```python
from build123d import *

# Parameters (mm, degrees)
F0_R     = 3.175
F1_DEPTH = 25.4


with BuildPart() as f1:
    # F0 (on Top) → F1 (new body)
    with BuildSketch(Plane.XY):
        with BuildLine():
            ThreePointArc((6.2681930411, -1.016), (6.3295152188, -0.5096440862), (6.35, 0))
            ThreePointArc((6.35, 0), (6.3295152188, 0.5096440862), (6.2681930411, 1.016))
            Line((6.2681930411, 1.016), (5.7634121265, 1.016))
            Line((5.7634121265, 1.016), (5.176824253, 0))
            Line((5.176824253, 0), (5.7634121265, -1.016))
            Line((5.7634121265, -1.016), (6.2681930411, -1.016))
        make_face()
        with BuildLine():
            ThreePointArc((6.2681930411, 1.016), (6.3295152188, 0.5096440862), (6.35, 0))
            ThreePointArc((6.35, 0), (6.3295152188, -0.5096440862), (6.2681930411, -1.016))
            Line((6.2681930411, -1.016), (6.9365878735, -1.016))
            Line((6.9365878735, -1.016), (7.523175747, 0))
            Line((7.523175747, 0), (6.9365878735, 1.016))
            Line((6.9365878735, 1.016), (6.2681930411, 1.016))
        make_face()
        with BuildLine():
            Line((5.7634121265, 1.016), (6.2681930411, 1.016))
            ThreePointArc((6.2681930411, 1.016), (4.4901280605, 4.4901280605), (1.016, 6.2681930411))
            Line((1.016, 6.2681930411), (1.016, 5.7634121265))
            Line((1.016, 5.7634121265), (0, 5.176824253))
            Line((0, 5.176824253), (-1.016, 5.7634121265))
            Line((-1.016, 5.7634121265), (-1.016, 6.2681930411))
            ThreePointArc((-1.016, 6.2681930411), (-4.4901280605, 4.4901280605), (-6.2681930411, 1.016))
            Line((-6.2681930411, 1.016), (-5.7634121265, 1.016))
            Line((-5.7634121265, 1.016), (-5.176824253, 0))
            Line((-5.176824253, 0), (-5.7634121265, -1.016))
            Line((-5.7634121265, -1.016), (-6.2681930411, -1.016))
            ThreePointArc((-6.2681930411, -1.016), (-4.4901280605, -4.4901280605), (-1.016, -6.2681930411))
            Line((-1.016, -6.2681930411), (-1.016, -5.7634121265))
            Line((-1.016, -5.7634121265), (0, -5.176824253))
            Line((0, -5.176824253), (1.016, -5.7634121265))
            Line((1.016, -5.7634121265), (1.016, -6.2681930411))
            ThreePointArc((1.016, -6.2681930411), (4.4901280605, -4.4901280605), (6.2681930411, -1.016))
            Line((6.2681930411, -1.016), (5.7634121265, -1.016))
            Line((5.7634121265, -1.016), (5.176824253, 0))
            Line((5.176824253, 0), (5.7634121265, 1.016))
        make_face()
        Circle(F0_R, mode=Mode.SUBTRACT)
        with BuildLine():
            Line((1.016, 5.7634121265), (1.016, 6.2681930411))
            ThreePointArc((1.016, 6.2681930411), (0, 6.35), (-1.016, 6.2681930411))
            Line((-1.016, 6.2681930411), (-1.016, 5.7634121265))
            Line((-1.016, 5.7634121265), (0, 5.176824253))
            Line((0, 5.176824253), (1.016, 5.7634121265))
        make_face()
        with BuildLine():
            ThreePointArc((-1.016, 6.2681930411), (0, 6.35), (1.016, 6.2681930411))
            Line((1.016, 6.2681930411), (1.016, 6.9365878735))
            Line((1.016, 6.9365878735), (0, 7.523175747))
            Line((0, 7.523175747), (-1.016, 6.9365878735))
            Line((-1.016, 6.9365878735), (-1.016, 6.2681930411))
        make_face()
        with BuildLine():
            Line((1.016, -6.9365878735), (1.016, -6.2681930411))
            ThreePointArc((1.016, -6.2681930411), (0, -6.35), (-1.016, -6.2681930411))
            Line((-1.016, -6.2681930411), (-1.016, -6.9365878735))
            Line((-1.016, -6.9365878735), (0, -7.523175747))
            Line((0, -7.523175747), (1.016, -6.9365878735))
        make_face()
        with BuildLine():
            ThreePointArc((-1.016, -6.2681930411), (0, -6.35), (1.016, -6.2681930411))
            Line((1.016, -6.2681930411), (1.016, -5.7634121265))
            Line((1.016, -5.7634121265), (0, -5.176824253))
            Line((0, -5.176824253), (-1.016, -5.7634121265))
            Line((-1.016, -5.7634121265), (-1.016, -6.2681930411))
        make_face()
        with BuildLine():
            Line((-5.7634121265, 1.016), (-6.2681930411, 1.016))
            ThreePointArc((-6.2681930411, 1.016), (-6.35, 0), (-6.2681930411, -1.016))
            Line((-6.2681930411, -1.016), (-5.7634121265, -1.016))
            Line((-5.7634121265, -1.016), (-5.176824253, 0))
            Line((-5.176824253, 0), (-5.7634121265, 1.016))
        make_face()
        with BuildLine():
            ThreePointArc((-6.2681930411, -1.016), (-6.35, 0), (-6.2681930411, 1.016))
            Line((-6.2681930411, 1.016), (-6.9365878735, 1.016))
            Line((-6.9365878735, 1.016), (-7.523175747, 0))
            Line((-7.523175747, 0), (-6.9365878735, -1.016))
            Line((-6.9365878735, -1.016), (-6.2681930411, -1.016))
        make_face()
    extrude(amount=F1_DEPTH)


solid = f1.part
```
Verification items for the finished model (mm, model axes). Round coordinates to 2 decimals unless told otherwise and drop trailing zeros. Order: outer loops, then holes, each group sorted by start corner. A loop starts at its lowest first (then second) coordinate and runs counter-clockwise, first axis right, second up. Notation, with made-up numbers: (16, 82) - (27, 82) arc R12 ccw to (27, 88) - close; hole circle Ø11 at (-15, 52). An arc over 180 degrees is marked (long way). Use CSV: the item, a comma, the result in double quotes. Start each with the question number.
1) Mould release check, pull along Y, two halves, no side actions. Record for faces 1 (the cylindrical face through (-0.69, -3.1, 12.52)), 2 (the flat face through (7.234, 0.501, 12.522)), 3 (the cylindrical face through (4.45, -4.53, 12.52)), 4 (the flat face through (-3.4, 0.1, 0)): +Y half, -Y half, draft (parallel to the pull), parting line (faces both ways), or undercut.
2) Thickness scan on L1, parallel to X at y = -2.5, z = 19; L2, parallel to Y at x = -1.5, z = 17.75; L3, parallel to X at y = -1.25, z = 18. Record the ranges inside material, lowest first.
3) Go/stop test with flat-tipped pins: P1, Ø6, axis at x = -3, y = -1.5, coming from the -Z side; P2, Ø3, axis at y = 2, z = 12, coming from the -X side; P3, Ø5, axis at x = -4.5, z = 9, coming from the +Y side; P4, Ø5, axis at y = 5.5, z = 12.5, coming from the +X side. Record where each tip stops, or that it passes through.
4) Section check A-A, the plane z = 3.5. Record the cut outline in (x, y) (3 decimals).
5) Section check D-D, the plane y = 5.75. Record the cut outline in (x, z).
6) Section check C-C, the plane y = -2.75. Record the cut outline in (x, z), plus the area to 3 significant figures.
7) Section check B-B, the plane x = 2.25. Record the cut outline in (y, z), plus the area to 3 significant figures.
Answers:
1,face 1,"undercut"
1,face 2,"+Y half"
1,face 3,"-Y half"
1,face 4,"draft"
2,L1,"x = -5.84 to -1.96, 1.96 to 5.84"
2,L2,"y = -6.17 to -2.8, 2.8 to 6.17"
2,L3,"x = -6.23 to -2.92, 2.92 to 6.23"
3,P1,"stops at z = 0"
3,P2,"stops at x = -7.23"
3,P3,"stops at y = 6.03"
3,P4,"stops at x = 5.6"
4,outline,"(-7.523, 0) - (-6.937, -1.016) - (-6.268, -1.016) arc R6.35 ccw to (-1.016, -6.268) - (-1.016, -6.937) - (0, -7.523) - (1.016, -6.937) - (1.016, -6.268) arc R6.35 ccw to (6.268, -1.016) - (6.937, -1.016) - (7.523, 0) - (6.937, 1.016) - (6.268, 1.016) arc R6.35 ccw to (1.016, 6.268) - (1.016, 6.937) - (0, 7.523) - (-1.016, 6.937) - (-1.016, 6.268) arc R6.35 ccw to (-6.268, 1.016) - (-6.937, 1.016) - close; hole circle Ø6.35 at (0, 0)"
5,outline,"(-2.69, 0) - (2.69, 0) - (2.69, 25.4) - (-2.69, 25.4) - close"
6,outline,"(-5.72, 0) - (-1.59, 0) - (-1.59, 25.4) - (-5.72, 25.4) - close; (1.59, 0) - (5.72, 0) - (5.72, 25.4) - (1.59, 25.4) - close"
6,area,"210 mm²"
7,outline,"(-5.94, 0) - (-2.24, 0) - (-2.24, 25.4) - (-5.94, 25.4) - close; (2.24, 0) - (5.94, 0) - (5.94, 25.4) - (2.24, 25.4) - close"
7,area,"188 mm²"
